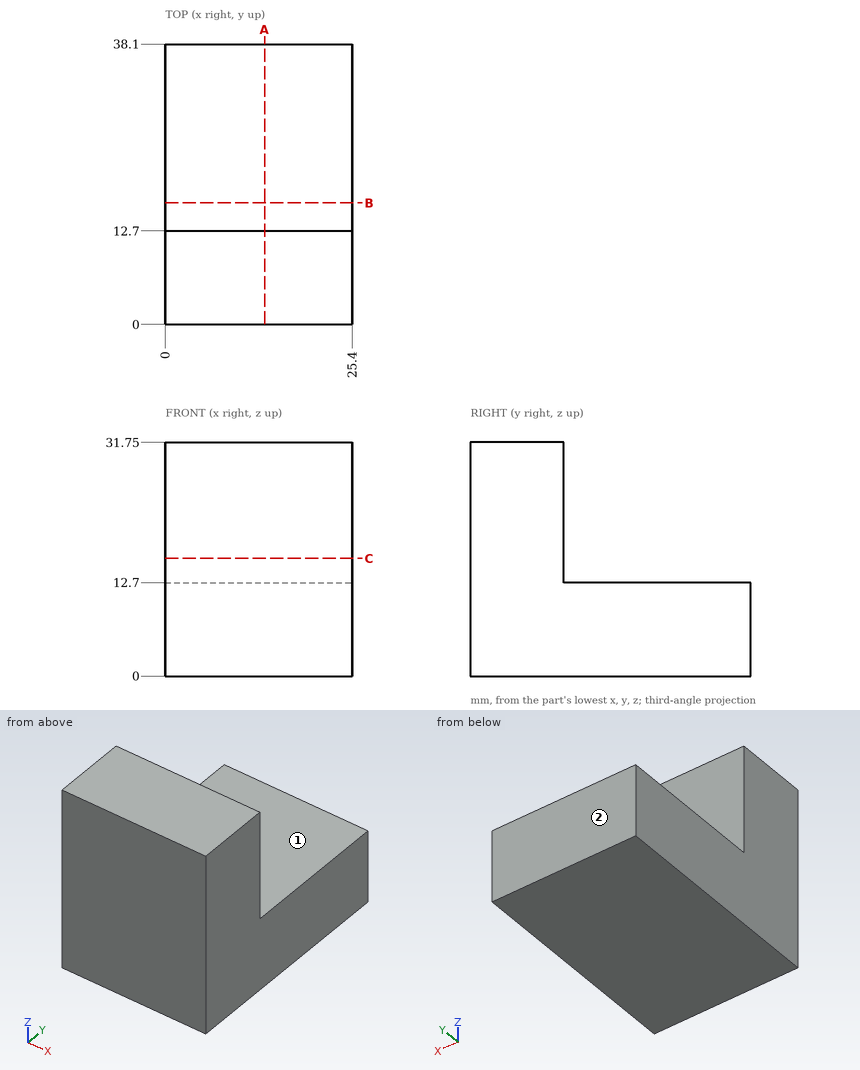
Verification items for this drawing (mm, ordinates from the low corner). A direction names the side the tool comes from. Coordinates: 2 decimals unless noted, no trailing zeros. Order: outer loops, then holes, each group sorted by start corner. A loop starts at its lowest first (then second) coordinate and runs counter-clockwise, first axis right, second up.
Q1. Sectioned sample at B-B on y = 16.5. Record the cut outline in (x, z), and give its area (3 significant figures).
Reply:
outline: (0, 0) - (25.4, 0) - (25.4, 12.7) - (0, 12.7) - close
area: 323 mm2
Q2. Thickness scan on probe 1 along Z at (x, y) = (23, 34.5). Record the ranges inside material, lowest first.
Reply:
probe 1: z = 0 to 12.7
Q3. Tool access check on the marked faces 1 and 2. Record the directions out of +Z, -Z, +X, -X, +Y, -Y that give a thin tool (end or side, any length) a straight path to the whole face; none if there is none.
Reply:
face 1: +Z, +X, -X, +Y
face 2: +Z, -Z, +X, -X, +Y
Q4. Depth check by flat-ended pin: pin 1 Ø12.5 at (x, y) = (11.5, 26) entering from +Z. Enter the tip coordinate at first touch or a pass-through.
Reply:
pin 1: stops at z = 12.7
Q5. Sectioned sample at A-A on x = 13.5. Record the cut outline in (y, z).
Reply:
outline: (0, 0) - (38.1, 0) - (38.1, 12.7) - (12.7, 12.7) - (12.7, 31.75) - (0, 31.75) - close
